Work out the finished part from the listing and answer in its coordinate system (mm). A direction names the side the tool comes from. Round coordinates to 2 decimals unless told otherwise and drop trailing zeros. Order: outer loops, then holes, each group sorted by start corner. A loop starts at its lowest first (then second) coordinate and runs counter-clockwise, first axis right, second up. Notation, with made-up numbers: (-28.5, 29.5) -> (9.5, 29.5) arc R9 ccw to (9.5, 43.5) -> close; hole circle Ø7 at (45.25, -26.5). An arc over 180 degrees is marked (long way). Use a Markdown table: item, result. Add a question column.
Item 1: A cutting plane is placed at B-B, the plane z = 17.75. Determine the outline of the cut face in (x, y).
Item 2: Find the intervals of material crossed by L1, parallel to X at y = -11, z = 13; L2, parallel to Y at x = 5, z = 18; L3, parallel to Z at x = 6.5, y = 8.25, in increasing order. Write a range as [from, to].
Item 3: Flat-ended cylindrical pins translate along their axes: P1, Ø2, axis at x = 2.5, y = -1, coming from the -Z side; P2, Ø3, axis at x = 5.5, y = -13, coming from the -Z side; P3, Ø8, axis at x = 6.5, z = 2.5, coming from the +Y side. Find the tip coordinate at first contact, or state that the pin passes through.
Item 4: A cutting plane is placed at D-D, the plane x = 7.25. Determine the outline of the cut face in (y, z).
Item 5: A cutting plane is placed at A-A, the plane z = 4.75. Determine the outline of the cut face in (x, y).
Item 6: For a pull along Z with two mould halves and no side action, classify faces 4 (the flat face through (-10.8, -0.2, 0.5)), 5 (the conical face through (12.653, 13.253, 0.135)), 6 (the flat face through (-12.8, 0, 9)), 7 (the flat face through (9.8, 0.2, 19)) as +Z half, -Z half, draft (parallel to the pull), parting line (faces both ways), or undercut.
Item 7: A tool of negligible diameter and unlimited length cuts with its end or side. For faces 1 (the flat face through (0, 0, 22)), 2 (the cylindrical face through (13.1, 13.26, 9.88)), 3 (the flat face through (11.82, 0.21, 2.01)), from which of +Z, -Z, +X, -X, +Y, -Y can it reach the whole face along a straight path? Write none if from no direction.
from build123d import *

# Parameters (mm, degrees)
PAD_DEPTH       = 15
CHAMFER_SIZE    = 1.99
CHAMFER001_SIZE = 6
SKETCH001_W     = 27.6
SKETCH001_H     = 7
PAD001_DEPTH    = 4
SKETCH002_W     = 31.6
SKETCH002_H     = 34
POCKET_DEPTH    = 23.001
FILLET_R        = 4
CHAMFER002_SIZE = 0.5


with BuildPart() as part:
    # Sketch → Pad (new body, symmetric)
    with BuildSketch(Plane.XZ):
        Polygon((-10.8, 0), (-10.8, 1), (-12.8, 1), (-12.8, 22), (12.8, 22), (12.8, 1), (10.8, 1), (10.8, 0), (13.8, 0), (13.8, 23), (-13.8, 23), (-13.8, 0), align=None)
    extrude(amount=PAD_DEPTH, both=True)

    # Chamfer
    chamfer_edges = [part.edges().sort_by_distance(p)[0] for p in [
        (-12.8, 0, 1),
        (12.8, 0, 1),
    ]]
    chamfer(chamfer_edges, length=CHAMFER_SIZE)

    # Chamfer001
    chamfer001_edges = [part.edges().sort_by_distance(p)[0] for p in [
        (12.8, 0, 22),
        (-12.8, 0, 22),
    ]]
    chamfer(chamfer001_edges, length=CHAMFER001_SIZE)

    # Sketch001 (on Face1 of Chamfer001) → Pad001 (join)
    with BuildSketch(Plane(origin=(0, 15, 0), x_dir=(1, 0, 0), z_dir=(0, 1, 0))):
        with Locations((0, -19.5)):
            Rectangle(SKETCH001_W, SKETCH001_H)
    pad001 = extrude(amount=-PAD001_DEPTH)

    # Mirrored: Pad001 across XZ
    add(pad001.mirror(Plane.XZ))

    # Sketch002 (on Face21 of Mirrored) → Pocket (cut, through all)
    with BuildSketch(Plane(origin=(0, 0, 23), x_dir=(-1, 0, 0), z_dir=(0, 0, 1))):
        Rectangle(SKETCH002_W, SKETCH002_H)
        with BuildLine():
            Line((-13.8, 11), (-13.8, -11))
            ThreePointArc((-13.8, -11), (-12.628427, -13.828427), (-9.8, -15))
            Line((-9.8, -15), (9.8, -15))
            ThreePointArc((9.8, -15), (12.628427, -13.828427), (13.8, -11))
            Line((13.8, -11), (13.8, 11))
            ThreePointArc((13.8, 11), (12.628427, 13.828427), (9.8, 15))
            Line((9.8, 15), (-9.8, 15))
            ThreePointArc((-9.8, 15), (-12.628427, 13.828427), (-13.8, 11))
        make_face(mode=Mode.SUBTRACT)
    extrude(amount=-POCKET_DEPTH, mode=Mode.SUBTRACT)

    # Fillet
    fillet_edges = [part.edges().sort_by_distance(p)[0] for p in [
        (0, 15, 23),
        (12.628427, 13.828427, 23),
        (13.8, 0, 23),
        (12.628427, -13.828427, 23),
        (0, -15, 23),
        (-12.628427, -13.828427, 23),
        (-13.8, 0, 23),
        (-12.628427, 13.828427, 23),
    ]]
    fillet(fillet_edges, radius=FILLET_R)

    # Chamfer002
    chamfer002_edges = [part.edges().sort_by_distance(p)[0] for p in [
        (13.8, 0, 0),
        (-13.8, 0, 0),
    ]]
    chamfer(chamfer002_edges, length=CHAMFER002_SIZE)


solid = part.part
Reported:
| question | item | result |
|---|---|---|
| 1 | outline | (-13.8, -11) arc R4 ccw to (-9.8, -15) -> (9.8, -15) arc R4 ccw to (13.8, -11) -> (13.8, 11) arc R4 ccw to (9.8, 15) -> (-9.8, 15) arc R4 ccw to (-13.8, 11) -> close; hole (-11.05, -11) -> (11.05, -11) -> (11.05, 11) -> (-11.05, 11) -> close |
| 2 | L1 | [-13.8, -12.8], [12.8, 13.8] |
| 2 | L2 | [-15, -11], [11, 15] |
| 2 | L3 | [22, 23] |
| 3 | P1 | z = 22 |
| 3 | P2 | z = 16 |
| 3 | P3 | through |
| 4 | outline | (-15, 16) -> (-11, 16) -> (-11, 21.55) -> (11, 21.55) -> (11, 16) -> (15, 16) -> (15, 19) arc R4 ccw to (11, 23) -> (-11, 23) arc R4 ccw to (-15, 19) -> close |
| 5 | outline | (-13.8, -11) arc R4 ccw to (-12.8, -13.65) -> (-12.8, 13.65) arc R4 ccw to (-13.8, 11) -> close; (12.8, -13.65) arc R4 ccw to (13.8, -11) -> (13.8, 11) arc R4 ccw to (12.8, 13.65) -> close |
| 6 | face 4 | draft |
| 6 | face 5 | -Z half |
| 6 | face 6 | undercut |
| 6 | face 7 | undercut |
| 7 | face 1 | -Z |
| 7 | face 2 | +Z, -Z, +X, +Y |
| 7 | face 3 | +Y, -Y |
